```python
from build123d import *

# Parameters (mm, degrees)
BOSS_EXTRUDE1_DEPTH     = 5
SKETCH2_R               = 1.5
CUT_EXTRUDE1_DEPTH      = 10
SKETCH4_W               = 6
SKETCH4_H               = 10.5
BOSS_EXTRUDE2_DEPTH     = 8
SKETCH3_W               = 5.5
SKETCH3_H               = 3
CUT_EXTRUDE2_DEPTH      = 27.379590534
CUT_EXTRUDE4_DEPTH      = 27.379590534
CUT_EXTRUDE4_DEPTH_BACK = 27.379590534
SKETCH9_W               = 6
SKETCH9_H               = 2.25
CUT_EXTRUDE5_DEPTH      = 5


with BuildPart() as part:
    # Sketch1 → Boss-Extrude1 (new body)
    with BuildSketch(Plane.XY):
        Polygon((0, 8.178190311), (0, 0), (23, 0), (23, 6), align=None)
    extrude(amount=BOSS_EXTRUDE1_DEPTH)

    # Sketch2 → Cut-Extrude1 (cut)
    with BuildSketch(Plane(origin=(0, 0, 0), x_dir=(-1, 0, 0), z_dir=(0, -1, 0))):
        with Locations(Location((-15, -2.5, 0), (0, 0, 90))):
            Circle(SKETCH2_R)
        with Locations(Location((-5, -2.5, 0), (0, 0, 90))):
            Circle(SKETCH2_R)
    extrude(amount=-CUT_EXTRUDE1_DEPTH, mode=Mode.SUBTRACT)

    # Sketch4 → Boss-Extrude2 (add)
    with BuildSketch(Plane(origin=(0, 0, 0), x_dir=(-1, 0, 0), z_dir=(0, -1, 0))):
        Polygon((0, -5), (-23, -5), (-23, -10), (14, -10), (14, 5), (-23, 5), (-23, 0), (0, 0), align=None)
        with Locations((8, -2.5)):
            Rectangle(SKETCH4_W, SKETCH4_H, mode=Mode.SUBTRACT)
    extrude(amount=-BOSS_EXTRUDE2_DEPTH)

    # Sketch3 → Cut-Extrude2 (cut, through all)
    with BuildSketch(Plane.XY.offset(5)):
        with Locations((5, 3.5)):
            Rectangle(SKETCH3_W, SKETCH3_H)
        with Locations((15, 3.5)):
            Rectangle(SKETCH3_W, SKETCH3_H)
    extrude(amount=-CUT_EXTRUDE2_DEPTH, mode=Mode.SUBTRACT)

    # Sketch5 → Cut-Extrude4 (cut, two sides: drawn at the far end of the back side and taken through both)
    with BuildSketch(Plane.XY.offset(5).offset(-CUT_EXTRUDE4_DEPTH_BACK)):
        Polygon((23, 8), (1.881551454, 8), (23, 6), align=None)
        Polygon((1.881551454, 8), (0, 8.178190311), (0, 8), align=None)
    extrude(amount=CUT_EXTRUDE4_DEPTH + CUT_EXTRUDE4_DEPTH_BACK, mode=Mode.SUBTRACT)

    # Sketch9 → Cut-Extrude5 (cut)
    with BuildSketch(Plane(origin=(0, 8, 0), x_dir=(1, 0, 0), z_dir=(0, 1, 0))):
        with Locations((-8, -8.875)):
            Rectangle(SKETCH9_W, SKETCH9_H)
    extrude(amount=-CUT_EXTRUDE5_DEPTH, mode=Mode.SUBTRACT)


solid = part.part
```
Part model, mm, in its own coordinate system. A direction names the side the tool comes from. Round coordinates to 2 decimals unless told otherwise and drop trailing zeros. Write each loop counter-clockwise with the first axis right and the second up, starting at its lowest first coordinate (ties: lowest second). Pieces come first, ordered by that corner, then holes.
Item 1: Cut at D-D, the plane x = 5. Give the cut face in (y, z), plus the area to 3 significant figures.
Results:
outline: (0, -5) - (2, -5) - (2, 1) - (0, 1) - close; (0, 4) - (2, 4) - (2, 5) - (5, 5) - (5, 4) - (7.7, 4) - (7.7, 10) - (0, 10) - close; (5, -5) - (7.7, -5) - (7.7, 1) - (5, 1) - close
area: 71.5 mm2
Item 2: Which spindle directions (+Z, -Z, +X, -X, +Y, -Y) get a long thin tool onto all of the face, cutting with end or side? Do faces 1 (the flat face through (4.8, 0, 0.7)), 2 (the flat face through (-5, 4, 4)), 3 (the flat face through (7.75, 3, 0)), 4 (the flat face through (-8, 4, -2.75)). Say none if no direction does.
Results:
face 1: +Z, -Z, +X, -X, -Y
face 2: +Y
face 3: -Z
face 4: +Y, -Y
Item 3: Two-plate mould, pull along X, no slides. Class faces 5 (the flat face through (-4, 8, 2)), 6 (the flat face through (15, 4, 5)), 7 (the flat face through (23, 3, 2)): +X half, -X half, draft (parallel to the pull), parting line (faces both ways), or undercut.
Results:
face 5: draft
face 6: undercut
face 7: +X half
Item 4: Cut at C-C, the plane z = 7.25. Give the cut face in (x, y).
Results:
outline: (-14, 0) - (-11, 0) - (-11, 8) - (-14, 8) - close; (-5, 0) - (23, 0) - (23, 6) - (1.88, 8) - (-5, 8) - close
Item 5: Cut at A-A, the plane z = -0.75. Give the cut face in (x, y).
Results:
outline: (-14, 0) - (-11, 0) - (-11, 8) - (-14, 8) - close; (-5, 0) - (23, 0) - (23, 6) - (1.88, 8) - (-5, 8) - close; hole (2.25, 2) - (7.75, 2) - (7.75, 5) - (2.25, 5) - close; hole (12.25, 2) - (17.75, 2) - (17.75, 5) - (12.25, 5) - close
Item 6: Drop flat-ended pins along their axis: pin 1 Ø3.5 at (x, z) = (15, 2.5) entering from +Y; pin 2 Ø1.1 at (x, z) = (-9, 8.5) entering from +Y; pin 3 Ø0.9 at (x, y) = (4, 3.5) entering from -Z. Give the stop position or say it passes through.
Results:
pin 1: stops at y = 6.92
pin 2: stops at y = 3
pin 3: stops at z = 5
Item 7: Probe L1, parallel to X at y = 0.75, z = 2.5; L2, parallel to X at y = 4, z = 6.75; L3, parallel to Z at x = 5, y = 6.15. List the from-to ranges inside material, lowest first.
Results:
L1: x = -14 to -11, -5 to 3.5, 6.5 to 13.5, 16.5 to 23
L2: x = -14 to -11, -5 to 23
L3: z = -5 to 1, 4 to 10
Item 8: Cut at B-B, the plane x = -6. Give the cut face in (y, z), plus the area to 4 significant figures.
Results:
outline: (0, -5) - (8, -5) - (8, -2.75) - (0, -2.75) - close; (0, 7.75) - (3, 7.75) - (3, 10) - (0, 10) - close
area: 24.75 mm2
